Design review of the part built by this model. Coordinates are the model's own, in mm. A direction names the side the tool comes from. Round coordinates to 2 decimals unless told otherwise and drop trailing zeros. Write each loop counter-clockwise with the first axis right and the second up, starting at its lowest first coordinate (ties: lowest second). Pieces come first, ordered by that corner, then holes.
from build123d import *

# Parameters (mm, degrees)
SKETCH1_R           = 43
BOSS_EXTRUDE1_DEPTH = 15
SKETCH2_R           = 4
CUT_EXTRUDE1_DEPTH  = 63.633856659
SKETCH3_R           = 3.875
CUT_EXTRUDE2_DEPTH  = 63.633856659
SKETCH4_R           = 33.25
SKETCH4_R_2         = 28
CUT_EXTRUDE3_DEPTH  = 3
SKETCH5_R           = 1.75
CUT_EXTRUDE4_DEPTH  = 63.633856659
CIRPATTERN1_COUNT   = 4
CHAMFER1_SIZE       = 2
CHAMFER1_SIZE2      = 7.464101615
CHAMFER2_SIZE       = 0.5


with BuildPart() as part:
    # Sketch1 → Boss-Extrude1 (new body)
    with BuildSketch(Plane(origin=(0, 0, 0), x_dir=(1, 0, 0), z_dir=(0, 1, 0))):
        with Locations(Location((0, 0, 0), (0, 0, 270))):
            Circle(SKETCH1_R)
    extrude(amount=BOSS_EXTRUDE1_DEPTH)

    # Sketch2 → Cut-Extrude1 (cut, through all)
    with BuildSketch(Plane.XZ):
        with Locations(Location((20, 0, 0), (0, 0, 270))):
            Circle(SKETCH2_R)
        with Locations(Location((-20, 0, 0), (0, 0, 270))):
            Circle(SKETCH2_R)
    extrude(amount=-CUT_EXTRUDE1_DEPTH, mode=Mode.SUBTRACT)

    # Sketch3 → Cut-Extrude2 (cut, through all)
    with BuildSketch(Plane(origin=(0, 15, 0), x_dir=(1, 0, 0), z_dir=(0, 1, 0))):
        with Locations(Location((0, 0, 0), (0, 0, 270))):
            Circle(SKETCH3_R)
    extrude(amount=-CUT_EXTRUDE2_DEPTH, mode=Mode.SUBTRACT)

    # Sketch4 → Cut-Extrude3 (cut)
    with BuildSketch(Plane(origin=(0, 15, 0), x_dir=(1, 0, 0), z_dir=(0, 1, 0))):
        with Locations(Location((0, 0, 0), (0, 0, 270))):
            Circle(SKETCH4_R)
        with Locations(Location((0, 0, 0), (0, 0, 270))):
            Circle(SKETCH4_R_2, mode=Mode.SUBTRACT)
    extrude(amount=-CUT_EXTRUDE3_DEPTH, mode=Mode.SUBTRACT)

    # Sketch5 → Cut-Extrude4 (cut, through all)
    with BuildSketch(Plane.XZ):
        with Locations(Location((36.5, 0, 0), (0, 0, 270))):
            Circle(SKETCH5_R)
    cut_extrude4 = extrude(amount=-CUT_EXTRUDE4_DEPTH, mode=Mode.SUBTRACT)

    # CirPattern1: Cut-Extrude4 ×4 about axis
    cirpattern1_axis = Axis((0, 0, 0), (0, 1, 0))
    for i in range(1, CIRPATTERN1_COUNT):
        add(cut_extrude4.rotate(cirpattern1_axis, i * 360 / CIRPATTERN1_COUNT), mode=Mode.SUBTRACT)

    # Chamfer1
    chamfer1_edges = [part.edges().sort_by_distance(p)[0] for p in [
        (0, 0, -43),
    ]]
    chamfer1_side = [part.faces().sort_by_distance(p)[0] for p in [
        (0, 0, -41.783776336),
    ]]
    chamfer(chamfer1_edges, length=CHAMFER1_SIZE, length2=CHAMFER1_SIZE2, reference=chamfer1_side[0])

    # Chamfer2
    chamfer2_edges = [part.edges().sort_by_distance(p)[0] for p in [
        (-20, 0, 4),
        (0, 0, -3.875),
        (20, 15, 4),
        (20, 0, 4),
    ]]
    chamfer(chamfer2_edges, length=CHAMFER2_SIZE)


solid = part.part
1) For faces 1 (the face through (-27.334, 13.521, -6.07)), 2 (the face through (0.38, 7.4, -34.79)), list the 3-axis set-ups (+Z, -Z, +X, -X, +Y, -Y) from which the entire face can be reached by the end or side of a thin tool; tool diameter is ignored.
2) For line 1 along X through (y, z) = (12.25, 15); line 2 along Z through (x, y) = (1, 1.75); line 3 along X through (y, z) = (13.5, -37), list the stretches that pass through material, from the lowest coordinate up.
3) For P1, Ø3, axis at x = 7.5, y = 3.5, coming from the -Z side; P2, Ø6, axis at x = 0, y = 2.5, coming from the +Z side; P3, Ø5, axis at x = -16, y = 11.5, coming from the -Z side, all flat-tipped, find the tip position at first contact; note any pin that passes through.
4) Add section B-B on y = 8.5. State the section outline as (x, z) points (3 decimals).
5) Add section D-D on y = 2.5. State the section outline as (x, z) points (3 decimals).
6) Add section A-A on y = 13.5. Count the separate pieces of the cut face and the enclosed holes in it, and give its area (3 significant figures).
7) The part is to be moulded in two halves that separate along X. For faces 3 (the face through (-9.4, 15, -32.1)), 4 (the face through (-24, 12, -15)), 5 (the face through (29.061, 11.179, -31.693)), 6 (the face through (34.79, 7.4, 0.38)), say which applies: pulls with the +X half, pulls with the -X half, needs draft (parallel to the pull), parting line crosses it, or undercut.
Computed:
1. face 1: +Y
1. face 2: +Y, -Y
2. line 1: x = -40.3 to -29.67, -23.64 to 23.64, 29.67 to 40.3
2. line 2: z = -41.46 to -37.94, -35.06 to -3.74, 3.74 to 35.06, 37.94 to 41.46
2. line 3: x = -21.91 to -1.68, 1.68 to 21.91
3. P1: stops at z = -41.74
3. P2: stops at z = 42.47
3. P3: stops at z = -40.83
4. outline: circle Ø86 at (0, 0); hole circle Ø3.5 at (-36.5, 0); hole circle Ø8 at (-20, 0); hole circle Ø7.75 at (0, 0); hole circle Ø3.5 at (0, -36.5); hole circle Ø3.5 at (0, 36.5); hole circle Ø8 at (20, 0); hole circle Ø3.5 at (36.5, 0)
5. outline: circle Ø83.34 at (0, 0); hole circle Ø3.5 at (-36.5, 0); hole circle Ø8 at (-20, 0); hole circle Ø7.75 at (0, 0); hole circle Ø3.5 at (0, -36.5); hole circle Ø3.5 at (0, 36.5); hole circle Ø8 at (20, 0); hole circle Ø3.5 at (36.5, 0)
6. separate pieces: 2
6. enclosed holes: 8
6. area: 4,610 mm2
7. face 3: needs draft
7. face 4: undercut
7. face 5: parting line crosses it
7. face 6: undercut
